Here's the drawing with two shaded views (mm, measured from the low corner). I have some questions. Coordinates: 2 decimals unless noted, no trailing zeros. Write each loop counter-clockwise with the first axis right and the second up, starting at its lowest first coordinate (ties: lowest second). Pieces come first, ordered by that corner, then holes. Notation, with made-up numbers: (0.5, -36.75) - (5.5, -36.75) arc R38 ccw to (5.5, 1.25) - close; hole circle Ø3 at (86.5, 12). An arc over 180 degrees is marked (long way). Answer in a Markdown table with one row per item. Add a question column.
Item 1: Imagine slicing it at D-D (x = 19). Please give me the cut outline in (y, z) (1 decimal), plus the area to 3 significant figures.
Item 2: Imagine slicing it at C-C (z = 0.6). Please give me the cut outline in (x, y), plus the area to 3 significant figures.
Item 3: Imagine slicing it at A-A (x = 5). Please give me the cut outline in (y, z) (1 decimal), plus the area to 3 significant figures.
Item 4: Imagine slicing it at B-B (y = 8.25). Please give me the cut outline in (x, z) (1 decimal).
Item 5: If I drill on probe 1 along Y at (x, z) = (20.5, 0.85); probe 2 along X at (y, z) = (6.75, 2.55); probe 3 along X at (y, z) = (7.75, 2.5), over which ranges is the centre line in solid material (lowest first)? Write a range as from..to.
Item 6: We'd pull the mould along X, two halves only. Please class the marked faces 1, 2 and 3: +X half, -X half, draft (parallel to the pull), parting line (faces both ways), or undercut.
Item 7: I'm going to push a flat-ended pin straight in: pin 1 (5 mm diameter, centred on x = 5, y = 6.77, fed in from +Z) (3 decimals). Where does the tip first touch, or does it pass through?
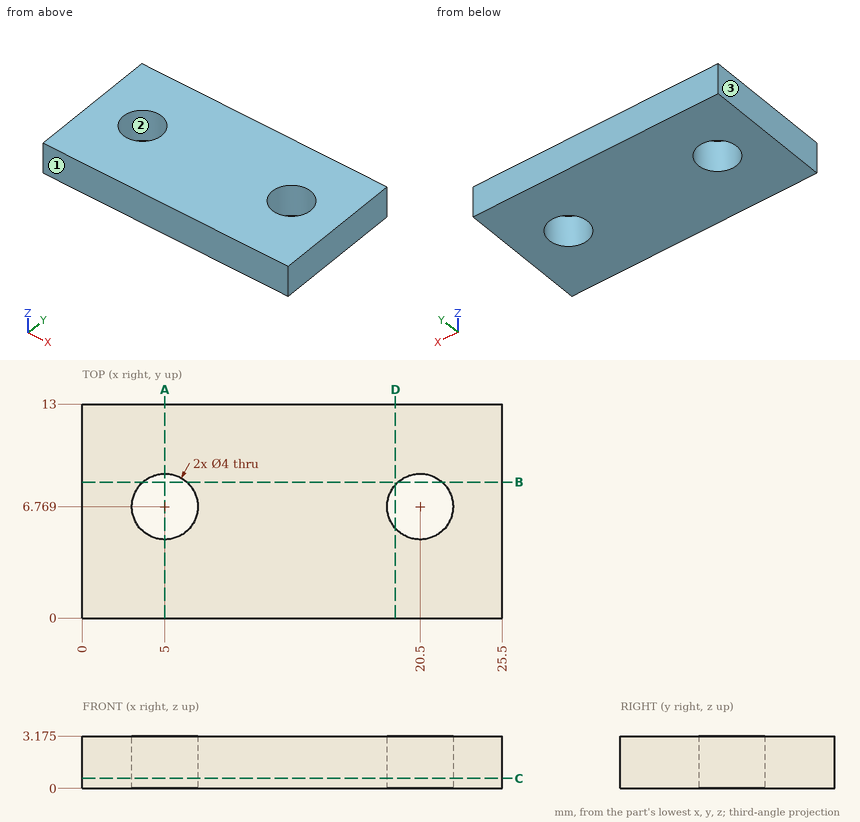
Here are the results:
| question | item | result |
|---|---|---|
| 1 | outline | (0, 0) - (5.4, 0) - (5.4, 3.2) - (0, 3.2) - close; (8.1, 0) - (13, 0) - (13, 3.2) - (8.1, 3.2) - close |
| 1 | area | 32.9 mm2 |
| 2 | outline | (0, 0) - (25.5, 0) - (25.5, 13) - (0, 13) - close; hole circle Ø4 at (5, 6.77); hole circle Ø4 at (20.5, 6.77) |
| 2 | area | 306 mm2 |
| 3 | outline | (0, 0) - (4.8, 0) - (4.8, 3.2) - (0, 3.2) - close; (8.8, 0) - (13, 0) - (13, 3.2) - (8.8, 3.2) - close |
| 3 | area | 28.6 mm2 |
| 4 | outline | (0, 0) - (3.7, 0) - (3.7, 3.2) - (0, 3.2) - close; (6.3, 0) - (19.2, 0) - (19.2, 3.2) - (6.3, 3.2) - close; (21.8, 0) - (25.5, 0) - (25.5, 3.2) - (21.8, 3.2) - close |
| 5 | probe 1 | y = 0..4.77, 8.77..13 |
| 5 | probe 2 | x = 0..3, 7..18.5, 22.5..25.5 |
| 5 | probe 3 | x = 0..3.26, 6.74..18.76, 22.24..25.5 |
| 6 | face 1 | draft |
| 6 | face 2 | undercut |
| 6 | face 3 | -X half |
| 7 | pin 1 | stops at z = 3.175 |
